Could you check a few things on this model? Use its own coordinates, in mm. Face numbers are marked on the shaded views. Round coordinates to 2 decimals unless told otherwise and drop trailing zeros. Loops run counter-clockwise (first coordinate to the right, second up) from the corner with the lowest first, then second, coordinate; pieces in that order, holes last.
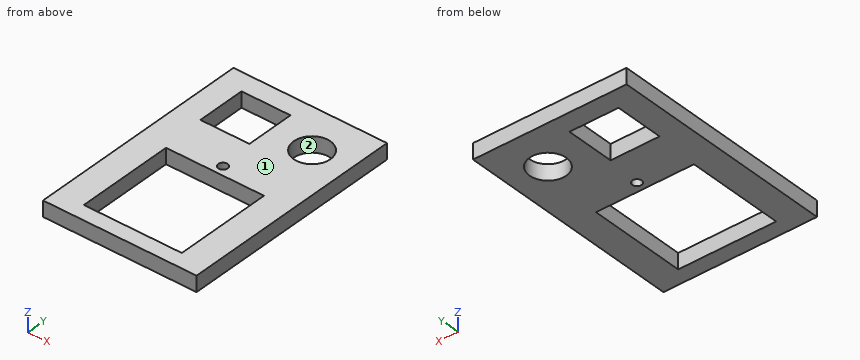
from build123d import *

# Parameters (mm, degrees)
F0_W     = 20
F0_H     = 20
F0_R     = 7.5
F1_DEPTH = 6.35


with BuildPart() as f1:
    # F0 (on Top) → F1 (new body)
    with BuildSketch(Plane.XY):
        Polygon((31.35, -46.35), (31.35, 46.35), (-31.35, 46.35), (-31.35, -46.35), (0, -46.35), align=None)
        Polygon((20, -40), (0, -40), (-20, -40), (-20, 0), (0, 0), (20, 0), align=None, mode=Mode.SUBTRACT)
        with Locations((-11.35, 28.35)):
            Rectangle(F0_W, F0_H, mode=Mode.SUBTRACT)
        with BuildLine():
            ThreePointArc((1.905, 3.905), (1.347038, 2.557962), (0, 2))
            ThreePointArc((0, 2), (-1.347038, 5.252038), (1.905, 3.905))
        make_face(mode=Mode.SUBTRACT)
        with Locations((15.85, 28.35)):
            Circle(F0_R, mode=Mode.SUBTRACT)
    extrude(amount=F1_DEPTH)


solid = f1.part
Item 1: We'd pull the mould along Y, two halves only. Please class the marked faces 1 and 2: released by +Y, released by -Y, zero draft, split by the parting line, or undercut.
Results list:
face 1: zero draft
face 2: undercut
Item 2: If we section it at B-B, the plane x = -19: Please give me the cut outline in (y, z).
Results list:
outline: (-46.35, 0) - (-40, 0) - (-40, 6.35) - (-46.35, 6.35) - close; (0, 0) - (18.35, 0) - (18.35, 6.35) - (0, 6.35) - close; (38.35, 0) - (46.35, 0) - (46.35, 6.35) - (38.35, 6.35) - close
Item 3: If we section it at D-D, the plane y = 32: Please give me the cut outline in (x, z).
Results list:
outline: (-31.35, 0) - (-21.35, 0) - (-21.35, 6.35) - (-31.35, 6.35) - close; (-1.35, 0) - (9.3, 0) - (9.3, 6.35) - (-1.35, 6.35) - close; (22.4, 0) - (31.35, 0) - (31.35, 6.35) - (22.4, 6.35) - close
Item 4: If we section it at C-C, the plane z = 3.25: Please give me the cut outline in (x, y) (3 decimals).
Results list:
outline: (-31.35, -46.35) - (31.35, -46.35) - (31.35, 46.35) - (-31.35, 46.35) - close; hole (-21.35, 18.35) - (-1.35, 18.35) - (-1.35, 38.35) - (-21.35, 38.35) - close; hole (-20, -40) - (20, -40) - (20, 0) - (-20, 0) - close; hole (0, 2) arc R1.905 ccw to (1.905, 3.905) arc R1.905 ccw (long way) to start; hole circle Ø15 at (15.85, 28.35)
Item 5: If I drill on line 1 along Y through (x, z) = (-7, 5.75); line 2 along Y through (x, z) = (0, 3.5); line 3 along X through (y, z) = (-38.5, 2.5), over which ranges is the centre line in solid material (lowest first)?
Results list:
line 1: y = -46.35 to -40, 0 to 18.35, 38.35 to 46.35
line 2: y = -46.35 to -40, 0 to 2, 5.81 to 46.35
line 3: x = -31.35 to -20, 20 to 31.35
Item 6: If we section it at A-A, the plane y = -37.5: Please give me the cut outline in (x, z), then the cut area to 3 significant figures.
Results list:
outline: (-31.35, 0) - (-20, 0) - (-20, 6.35) - (-31.35, 6.35) - close; (20, 0) - (31.35, 0) - (31.35, 6.35) - (20, 6.35) - close
area: 144 mm2
Item 7: Will this pin go through, and if not, where does the flat tip stop? pin 1 (3 mm diameter, centred on x = 0, y = 3.905, fed in from -Z).
Results list:
pin 1: passes through
